Here's the drawing with two shaded views (mm, measured from the low corner). I have some questions. A direction names the side the tool comes from. Round coordinates to 2 decimals unless told otherwise and drop trailing zeros. Loops run counter-clockwise (first coordinate to the right, second up) from the corner with the lowest first, then second, coordinate; pieces in that order, holes last. Notation, with made-up numbers: (82.5, 22.5) -> (105.5, 22.5) arc R20 cw to (105.5, 43.5) -> close; hole circle Ø2 at (-20, 58.5). An arc over 180 degrees is marked (long way). Use a Markdown table: item, result.
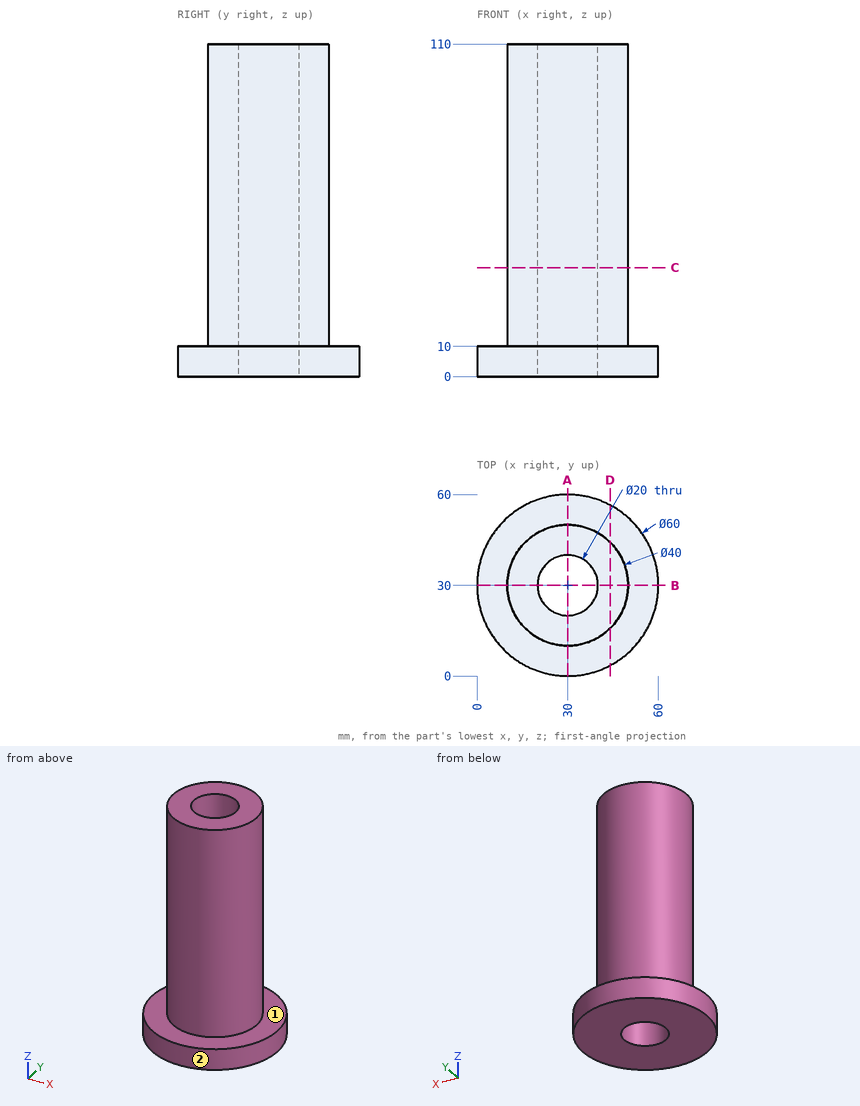
1. I want a section at D-D (x = 44). Please give me the cut outline in (y, z).
Answer sheet:
| item | result |
|---|---|
| outline | (3.47, 0) -> (56.53, 0) -> (56.53, 10) -> (44.28, 10) -> (44.28, 110) -> (15.72, 110) -> (15.72, 10) -> (3.47, 10) -> close |
2. I want a section at A-A (x = 30). Please give me the cut outline in (y, z).
Answer sheet:
| item | result |
|---|---|
| outline | (0, 0) -> (20, 0) -> (20, 110) -> (10, 110) -> (10, 10) -> (0, 10) -> close; (40, 0) -> (60, 0) -> (60, 10) -> (50, 10) -> (50, 110) -> (40, 110) -> close |
3. Will these pins go through, and if not, where does the flat tip stop? pin 1 Ø3 at (x, z) = (13, 29.5) entering from +Y; pin 2 Ø12 at (x, z) = (24.5, 75.5) entering from -Y; pin 3 Ø2 at (x, z) = (39.5, 17) entering from +Y.
Answer sheet:
| item | result |
|---|---|
| pin 1 | stops at y = 42.64 |
| pin 2 | stops at y = 10 |
| pin 3 | stops at y = 48.1 |
4. I need wall thicknesses on line 1 (Y direction, x = 30, z = 37); line 2 (Z direction, x = 19, y = 57.5); line 3 (Y direction, x = 37.5, z = 49.5). Which ranges of each line are inside material? Lowest first, please.
Answer sheet:
| item | result |
|---|---|
| line 1 | y = 10 to 20, 40 to 50 |
| line 2 | z = 0 to 10 |
| line 3 | y = 11.46 to 23.39, 36.61 to 48.54 |
5. I want a section at C-C (z = 36). Please give me the cut outline in (x, y), plus the area to 3 significant figures.
Answer sheet:
| item | result |
|---|---|
| outline | circle Ø40 at (30, 30); hole circle Ø20 at (30, 30) |
| area | 942 mm² |
6. Which directions (+Z, -Z, +X, -X, +Y, -Y) give clear straight access to the entire face, cutting with the end or side of a thin tool? Please do the marked faces 1 and 2.
Answer sheet:
| item | result |
|---|---|
| face 1 | +Z |
| face 2 | +Z, -Z |
